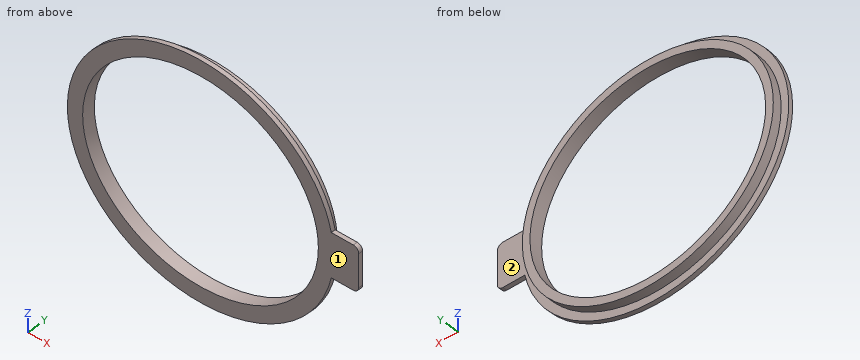
```python
from build123d import *

# Parameters (mm, degrees)
SKETCH1_RX          = 115
SKETCH1_RY          = 100
SKETCH1_RX_2        = 108
SKETCH1_RY_2        = 93
BOSS_EXTRUDE1_DEPTH = 12
SKETCH2_RX          = 122
SKETCH2_RY          = 107
SKETCH2_RX_2        = 108
SKETCH2_RY_2        = 93
BOSS_EXTRUDE2_DEPTH = 4
BOSS_EXTRUDE3_DEPTH = 4
FILLET1_R           = 5


with BuildPart() as part:
    # Sketch1 → Boss-Extrude1 (new body)
    with BuildSketch(Plane(origin=(0, 0, 0), x_dir=(1, 0, 0), z_dir=(0, 1, 0))):
        with Locations(Location((0, 0), (0, 0, 180))):
            Ellipse(SKETCH1_RX, SKETCH1_RY)
        with Locations((0, 0)):
            Ellipse(SKETCH1_RX_2, SKETCH1_RY_2, mode=Mode.SUBTRACT)
    extrude(amount=BOSS_EXTRUDE1_DEPTH)

    # Sketch2 → Boss-Extrude2 (add)
    with BuildSketch(Plane(origin=(0, 0, 0), x_dir=(1, 0, 0), z_dir=(0, 1, 0))):
        with Locations(Location((0, 0), (0, 0, 180))):
            Ellipse(SKETCH2_RX, SKETCH2_RY)
        with Locations(Location((0, 0), (0, 0, 180))):
            Ellipse(SKETCH2_RX_2, SKETCH2_RY_2, mode=Mode.SUBTRACT)
    extrude(amount=BOSS_EXTRUDE2_DEPTH)

    # Sketch3 → Boss-Extrude3 (add)
    with BuildSketch(Plane(origin=(0, 0, 0), x_dir=(1, 0, 0), z_dir=(0, 1, 0))):
        Polygon((115, -20), (145, -20), (145, 20), (115, 20), (115, 0), align=None)
    extrude(amount=BOSS_EXTRUDE3_DEPTH)

    # Fillet1
    fillet1_edges = [part.edges().sort_by_distance(p)[0] for p in [
        (145, 2, -20),
        (145, 2, 20),
    ]]
    fillet(fillet1_edges, radius=FILLET1_R)


solid = part.part
```
Design review of the part built by this model. Coordinates are the model's own, in mm. Face numbers are marked on the shaded views. A direction names the side the tool comes from. Coordinates: 2 decimals unless noted, no trailing zeros. One line per question, with ' | ' between items.
(1) Wall thickness on probe 1 along Z at (x, y) = (-4, 11); probe 2 along X at (y, z) = (9.75, 45); probe 3 along Z at (x, y) = (-55.5, 8.25): over which ranges is each line inside the solid? List them lowest first.
Filled in:
probe 1: z = -99.94 to -92.94, 92.94 to 99.94 | probe 2: x = -102.7 to -94.52, 94.52 to 102.7 | probe 3: z = -87.58 to -79.78, 79.78 to 87.58
(2) For pin 1 Ø1.2 at (x, y) = (133.5, 1.5) entering from +Z; pin 2 Ø5 at (y, z) = (2.5, 26.5) entering from +X; pin 3 Ø3 at (y, z) = (10.5, 53) entering from -X, all flat-tipped, find the tip position at first contact; note any pin that passes through.
Filled in:
pin 1: stops at z = 20 | pin 2: stops at x = 118.89 | pin 3: stops at x = -98.58
(3) Machinability: for the marked faces 1 and 2, which of the approach directions +Z, -Z, +X, -X, +Y, -Y give a long, thin tool a straight path to every point of the face, cutting with its end or side? Answer none if there is none.
Filled in:
face 1: +Z, -Z, +X, -X, -Y | face 2: +Y
